```python
from build123d import *

# Parameters (mm, degrees)
SKETCH1_W           = 60
SKETCH1_H           = 28
SKETCH1_R           = 4.25
BOSS_EXTRUDE1_DEPTH = 5
CUT_EXTRUDE1_DEPTH  = 35.583232932
CUT_EXTRUDE2_REACH  = 43.34
SKETCH3_R           = 1.75
FILLET1_R           = 5
FILLET2_R           = 2
SKETCH4_R           = 1.25
BOSS_EXTRUDE2_DEPTH = 3
SKETCH5_W           = 3.75
SKETCH5_H           = 8.5
SKETCH5_W_2         = 9.5
BOSS_EXTRUDE4_DEPTH = 10
SKETCH6_W           = 36
SKETCH6_H           = 8.5
CUT_EXTRUDE3_DEPTH  = 1
SKETCH7_R           = 1.75
CUT_EXTRUDE4_DEPTH  = 45.988887539
SKETCH8_R           = 2.1
CUT_EXTRUDE5_DEPTH  = 4
SKETCH9_R           = 2.1
CUT_EXTRUDE6_DEPTH  = 2
CHAMFER1_SIZE       = 0.5
CUT_EXTRUDE7_REACH  = 46.777
SKETCH10_W          = 2.5
SKETCH10_H          = 8.5
FILLET3_R           = 1.5
FILLET4_R           = 1


with BuildPart() as part:
    # Sketch1 → Boss-Extrude1 (new, symmetric)
    with BuildSketch(Plane.XY):
        Rectangle(SKETCH1_W, SKETCH1_H)
        with Locations((-22, 6)):
            Circle(SKETCH1_R, mode=Mode.SUBTRACT)
        with Locations((22, 6)):
            Circle(SKETCH1_R, mode=Mode.SUBTRACT)
    extrude(amount=BOSS_EXTRUDE1_DEPTH, both=True)

    # Sketch2 → Cut-Extrude1 (cut, through all)
    with BuildSketch(Plane(origin=(0, 0, -5), x_dir=(-1, 0, 0), z_dir=(0, 0, -1))):
        Polygon((8, -6.75), (3, -6.75), (3, 4.25), (4, 4.25), (4, 9.25), (7, 9.25), (7, 4.25), (8, 4.25), align=None)
        Polygon((-8, -6.75), (-8, 4.25), (-7, 4.25), (-7, 9.25), (-4, 9.25), (-4, 4.25), (-3, 4.25), (-3, -6.75), align=None)
    extrude(amount=-CUT_EXTRUDE1_DEPTH, mode=Mode.SUBTRACT)

    # Sketch3 → Cut-Extrude2 (cut, up to next)
    with BuildSketch(Plane(origin=(0, 14, 0), x_dir=(1, 0, 0), z_dir=(0, 1, 0)), mode=Mode.PRIVATE) as cut_extrude2_sk1:
        with Locations(Location((-22, 0, 0), (0, 0, 270))):
            Circle(SKETCH3_R)
    cut_extrude2_tool1 = extrude(cut_extrude2_sk1.sketch, amount=-CUT_EXTRUDE2_REACH, mode=Mode.PRIVATE) & part.part
    # Sketch3 → Cut-Extrude2 (cut, up to next)
    with BuildSketch(Plane(origin=(0, 14, 0), x_dir=(1, 0, 0), z_dir=(0, 1, 0)), mode=Mode.PRIVATE) as cut_extrude2_sk2:
        with Locations(Location((22, 0, 0), (0, 0, 270))):
            Circle(SKETCH3_R)
    cut_extrude2_tool2 = extrude(cut_extrude2_sk2.sketch, amount=-CUT_EXTRUDE2_REACH, mode=Mode.PRIVATE) & part.part
    add(cut_extrude2_tool1.solids().sort_by_distance((-22, 14, 0))[0], mode=Mode.SUBTRACT)
    add(cut_extrude2_tool2.solids().sort_by_distance((22, 14, 0))[0], mode=Mode.SUBTRACT)

    # Fillet1
    fillet1_edges = [part.edges().sort_by_distance(p)[0] for p in [
        (-30, 14, 0),
        (30, 14, 0),
        (30, -14, 0),
        (-30, -14, 0),
    ]]
    fillet(fillet1_edges, radius=FILLET1_R)

    # Fillet2
    # the kernel refuses this fillet: 2 mm, written as the material it adds along each edge
    with BuildSketch(Plane(origin=(-8, 4.25, -5), x_dir=(0, -1, 0), z_dir=(0, 0, 1)), Plane(origin=(3, 4.25, -5), x_dir=(0, -1, 0), z_dir=(0, 0, 1))) as fillet2_piece_1:
        with BuildLine():
            CenterArc((1.732050808, 2), FILLET2_R, 210, 60)
            Line((0, 1), (-0.034641016, 0.98))
            ThreePointArc((-0.034641016, 0.98), (-0.04, 0.5), (-0.04, 0))
            Line((-0.04, 0), (0, -0.04))
            Line((0, -0.04), (1.732050808, -0.04))
            Line((1.732050808, -0.04), (1.732050808, 0))
        make_face()
    extrude(amount=10)
    with BuildSketch(Plane(origin=(-3, 4.25, -5), x_dir=(-1, 0, 0), z_dir=(0, 0, 1)), Plane(origin=(8, 4.25, -5), x_dir=(-1, 0, 0), z_dir=(0, 0, 1))) as fillet2_piece_2:
        with BuildLine():
            CenterArc((2, 1.732050808), FILLET2_R, 180, 60)
            Line((0, 1.732050808), (-0.04, 1.732050808))
            Line((-0.04, 1.732050808), (-0.04, 0))
            Line((-0.04, 0), (0, -0.04))
            ThreePointArc((0, -0.04), (0.5, -0.04), (0.98, -0.034641016))
            Line((0.98, -0.034641016), (1, 0))
        make_face()
    extrude(amount=10)

    # Sketch4 → Boss-Extrude2 (add)
    with BuildSketch(Plane(origin=(0, 0, -5), x_dir=(-1, 0, 0), z_dir=(0, 0, -1))):
        with BuildLine():
            Line((-18, 14), (18, 14))
            Line((18, 14), (18, 29))
            ThreePointArc((18, 29), (17.121320344, 31.121320344), (15, 32))
            Line((15, 32), (-15, 32))
            ThreePointArc((-15, 32), (-17.121320344, 31.121320344), (-18, 29))
            Line((-18, 29), (-18, 14))
        make_face()
        with Locations((-13.85, 22.25)):
            Circle(SKETCH4_R, mode=Mode.SUBTRACT)
        with Locations((13.85, 22.25)):
            Circle(SKETCH4_R, mode=Mode.SUBTRACT)
        with BuildLine():
            Line((-11.65, 28.5), (11.65, 28.5))
            ThreePointArc((11.65, 28.5), (12.003553391, 28.353553391), (12.15, 28))
            Line((12.15, 28), (12.15, 16.5))
            ThreePointArc((12.15, 16.5), (12.003553391, 16.146446609), (11.65, 16))
            Line((11.65, 16), (-11.65, 16))
            ThreePointArc((-11.65, 16), (-12.003553391, 16.146446609), (-12.15, 16.5))
            Line((-12.15, 16.5), (-12.15, 28))
            ThreePointArc((-12.15, 28), (-12.003553391, 28.353553391), (-11.65, 28.5))
        make_face(mode=Mode.SUBTRACT)
    extrude(amount=-BOSS_EXTRUDE2_DEPTH)

    # Sketch5 → Boss-Extrude4 (add)
    with BuildSketch(Plane.XY.offset(5)):
        with Locations((-8.125, -2.5)):
            Rectangle(SKETCH5_W, SKETCH5_H)
        with Locations((0, -2.5)):
            Rectangle(SKETCH5_W_2, SKETCH5_H)
        with Locations((8.125, -2.5)):
            Rectangle(SKETCH5_W, SKETCH5_H)
    extrude(amount=-BOSS_EXTRUDE4_DEPTH)

    # Sketch6 → Cut-Extrude3 (cut)
    with BuildSketch(Plane.XY.offset(5)):
        with Locations((0, -2.5)):
            Rectangle(SKETCH6_W, SKETCH6_H)
    extrude(amount=-CUT_EXTRUDE3_DEPTH, mode=Mode.SUBTRACT)

    # Sketch7 → Cut-Extrude4 (cut, through all)
    with BuildSketch(Plane.XY.offset(5)):
        with Locations((25.5, -9.5)):
            Circle(SKETCH7_R)
        with Locations((-25.5, -9.5)):
            Circle(SKETCH7_R)
        with Locations((-12, 6)):
            Circle(SKETCH7_R)
        with Locations((12, 6)):
            Circle(SKETCH7_R)
    extrude(amount=-CUT_EXTRUDE4_DEPTH, mode=Mode.SUBTRACT)

    # Sketch8 → Cut-Extrude5 (cut)
    with BuildSketch(Plane(origin=(0, 0, 5), x_dir=(-1, 0, 0), z_dir=(0, 0, -1))):
        with Locations((-12, 6)):
            Circle(SKETCH8_R)
        with Locations((-25.5, -9.5)):
            Circle(SKETCH8_R)
        with Locations((25.5, -9.5)):
            Circle(SKETCH8_R)
        with Locations((12, 6)):
            Circle(SKETCH8_R)
    extrude(amount=CUT_EXTRUDE5_DEPTH, mode=Mode.SUBTRACT)

    # Sketch9 → Cut-Extrude6 (cut)
    with BuildSketch(Plane.XZ.offset(-14)):
        with Locations(Location((-22, 0, 0), (0, 0, 270))):
            Circle(SKETCH9_R)
        with Locations(Location((22, 0, 0), (0, 0, 270))):
            Circle(SKETCH9_R)
    extrude(amount=CUT_EXTRUDE6_DEPTH, mode=Mode.SUBTRACT)

    # Chamfer1
    # the kernel refuses this chamfer: 0.5 mm, written as the material it takes off along each edge
    with BuildSketch(Plane(origin=(-25.5, -9.5, 1), x_dir=(1, 0, 0), z_dir=(0, -1, 0))) as chamfer1_piece_1_section:
        Polygon((1.75, -CHAMFER1_SIZE), (1.75 + CHAMFER1_SIZE, 0), (1.75, 0), align=None)
    chamfer1_piece_1 = revolve(axis=Axis((-25.5, -9.5, 1), (0, 0, 1)), mode=Mode.PRIVATE)
    chamfer1_piece_1 = chamfer1_piece_1 & Plane(origin=(-25.5, -9.5, 0.675956313), x_dir=(-1, 0, 0), z_dir=(0, 0, 1)) * Cylinder(2.1, 9, mode=Mode.PRIVATE)
    add(chamfer1_piece_1, mode=Mode.SUBTRACT)
    with BuildSketch(Plane(origin=(25.5, -9.5, 1), x_dir=(1, 0, 0), z_dir=(0, -1, 0))) as chamfer1_piece_2_section:
        Polygon((1.75, -CHAMFER1_SIZE), (1.75 + CHAMFER1_SIZE, 0), (1.75, 0), align=None)
    chamfer1_piece_2 = revolve(axis=Axis((25.5, -9.5, 1), (0, 0, 1)), mode=Mode.PRIVATE)
    chamfer1_piece_2 = chamfer1_piece_2 & Plane(origin=(25.5, -9.5, 0.675956313), x_dir=(-1, 0, 0), z_dir=(0, 0, 1)) * Cylinder(2.1, 9, mode=Mode.PRIVATE)
    add(chamfer1_piece_2, mode=Mode.SUBTRACT)
    with BuildSketch(Plane(origin=(-22, 12, 0), x_dir=(0, 0, 1), z_dir=(-1, 0, 0))) as chamfer1_piece_3_section:
        Polygon((1.75, -CHAMFER1_SIZE), (1.75 + CHAMFER1_SIZE, 0), (1.75, 0), align=None)
    chamfer1_piece_3 = revolve(axis=Axis((-22, 12, 0), (0, 1, 0)), mode=Mode.PRIVATE)
    chamfer1_piece_3 = chamfer1_piece_3 & Plane(origin=(-22, 11.675956313, 0), x_dir=(0, 0, -1), z_dir=(0, 1, 0)) * Cylinder(2.1, 9, mode=Mode.PRIVATE)
    add(chamfer1_piece_3, mode=Mode.SUBTRACT)
    with BuildSketch(Plane(origin=(22, 12, 0), x_dir=(0, 0, 1), z_dir=(-1, 0, 0))) as chamfer1_piece_4_section:
        Polygon((1.75, -CHAMFER1_SIZE), (1.75 + CHAMFER1_SIZE, 0), (1.75, 0), align=None)
    chamfer1_piece_4 = revolve(axis=Axis((22, 12, 0), (0, 1, 0)), mode=Mode.PRIVATE)
    chamfer1_piece_4 = chamfer1_piece_4 & Plane(origin=(22, 11.675956313, 0), x_dir=(0, 0, -1), z_dir=(0, 1, 0)) * Cylinder(2.1, 9, mode=Mode.PRIVATE)
    add(chamfer1_piece_4, mode=Mode.SUBTRACT)
    with BuildSketch(Plane(origin=(-12, 6, 1), x_dir=(1, 0, 0), z_dir=(0, -1, 0))) as chamfer1_piece_5_section:
        Polygon((1.75, -CHAMFER1_SIZE), (1.75 + CHAMFER1_SIZE, 0), (1.75, 0), align=None)
    chamfer1_piece_5 = revolve(axis=Axis((-12, 6, 1), (0, 0, 1)), mode=Mode.PRIVATE)
    chamfer1_piece_5 = chamfer1_piece_5 & Plane(origin=(-12, 6, 0.675956313), x_dir=(-1, 0, 0), z_dir=(0, 0, 1)) * Cylinder(2.1, 9, mode=Mode.PRIVATE)
    add(chamfer1_piece_5, mode=Mode.SUBTRACT)
    with BuildSketch(Plane(origin=(12, 6, 1), x_dir=(1, 0, 0), z_dir=(0, -1, 0))) as chamfer1_piece_6_section:
        Polygon((1.75, -CHAMFER1_SIZE), (1.75 + CHAMFER1_SIZE, 0), (1.75, 0), align=None)
    chamfer1_piece_6 = revolve(axis=Axis((12, 6, 1), (0, 0, 1)), mode=Mode.PRIVATE)
    chamfer1_piece_6 = chamfer1_piece_6 & Plane(origin=(12, 6, 0.675956313), x_dir=(-1, 0, 0), z_dir=(0, 0, 1)) * Cylinder(2.1, 9, mode=Mode.PRIVATE)
    add(chamfer1_piece_6, mode=Mode.SUBTRACT)

    # Sketch10 → Cut-Extrude7 (cut, up to next)
    with BuildSketch(Plane.XY.offset(4), mode=Mode.PRIVATE) as cut_extrude7_sk1:
        with Locations((-16.75, -2.5)):
            Rectangle(SKETCH10_W, SKETCH10_H)
    cut_extrude7_tool1 = extrude(cut_extrude7_sk1.sketch, amount=-CUT_EXTRUDE7_REACH, mode=Mode.PRIVATE) & part.part
    # Sketch10 → Cut-Extrude7 (cut, up to next)
    with BuildSketch(Plane.XY.offset(4), mode=Mode.PRIVATE) as cut_extrude7_sk2:
        with Locations((16.75, -2.5)):
            Rectangle(SKETCH10_W, SKETCH10_H)
    cut_extrude7_tool2 = extrude(cut_extrude7_sk2.sketch, amount=-CUT_EXTRUDE7_REACH, mode=Mode.PRIVATE) & part.part
    add(cut_extrude7_tool1.solids().sort_by_distance((-16.75, -2.5, 4))[0], mode=Mode.SUBTRACT)
    add(cut_extrude7_tool2.solids().sort_by_distance((16.75, -2.5, 4))[0], mode=Mode.SUBTRACT)

    # Fillet3
    fillet3_edges = [part.edges().sort_by_distance(p)[0] for p in [
        (-6.25, 1.75, -0.5),
        (-4.75, 1.75, -0.5),
        (4.75, 1.75, -0.5),
        (6.25, 1.75, -0.5),
        (6.25, -2.5, 4),
        (-6.25, -2.5, 4),
        (-4.75, -2.5, 4),
        (4.75, -2.5, 4),
        (-15.5, -2.5, 4),
        (15.5, -2.5, 4),
    ]]
    fillet(fillet3_edges, radius=FILLET3_R)

    # Fillet4
    fillet4_edges = [part.edges().sort_by_distance(p)[0] for p in [
        (-4, 4.25, 0),
        (-4, 9.25, 0),
        (-7, 9.25, 0),
        (-7, 4.25, 0),
        (7, 4.25, 0),
        (7, 9.25, 0),
        (4, 9.25, 0),
        (4, 4.25, 0),
    ]]
    fillet(fillet4_edges, radius=FILLET4_R)


solid = part.part
```
CAD build for the part. Positions are in the model's coordinates, mm. A direction names the side the tool comes from. Give positions to 0.01 mm unless a question says otherwise; leave off trailing zeros. Write each loop counter-clockwise with the first axis right and the second up, starting at its lowest first coordinate (ties: lowest second). Pieces come first, ordered by that corner, then holes. Notation, with made-up numbers: M -12,45 L 34,45 A21 cw 34,80 Z; hole C 32.5,5 d9. An arc over 180 degrees is marked long. Return JSON: item names as keys, results as strings. Group by question number.
(1) Band-saw the part on B-B (x = 22). Give the cut face in (y, z), and give its area (3 significant figures).
(2) Mould opens along Y. For faces 1 (the face through (0, 32, -4)), 2 (the face through (23.75, -9.42, -2.21)), 3 (the face through (-29, -12, 0)), 4 (the face through (-3.17, 3.32, -0.07)) say: pulls with the +Y half, pulls with the -Y half, needs draft (parallel to the pull), parting line crosses it, or undercut.
(3) Band-saw the part on A-A (y = -2.5). Give the cut face in (x, z).
(4) Flat gauge pins, fed straight in: pin 1 Ø2.5 at (y, z) = (21.5, -4) entering from -X; pin 2 Ø1 at (y, z) = (21.5, -3.5) entering from +X; pin 3 Ø5.5 at (x, y) = (12, 6) entering from -Z; pin 4 Ø8 at (x, y) = (-16.5, 18.5) entering from +Z. Where does each tip first touch, or does it go through?
(5) Drill centre lines: L1, parallel to Y at x = -22, z = -2.5; L2, parallel to X at y = -1, z = 2.75; L3, parallel to Y at x = 12, z = 2.25. Where is each one in solid material? Low to high. Write a range as [from, to].
(6) Band-saw the part on D-D (y = 6). State how many separate pieces and enclosed holes the cut face has, and give its area (3 significant figures).
(7) Band-saw the part on C-C (y = 22.25). Give the cut face in (x, z), and give its area (3 significant figures).
(8) 3-axis set-ups, long thin cutter, end or side, ignore diameter. For faces 5 (the face through (30, 0, 0)), 6 (the face through (3.18, 3.35, -0.07)): which of +Z, -Z, +X, -X, +Y, -Y reach the whole face in a straight line?
Entries:
{
 "1": {"outline": "M -14,-5 L 1.75,-5 L 1.75,5 L -14,5 Z; M 10.25,-5 L 14,-5 L 14,-2.1 L 11.85,-2.1 L 11.5,-1.75 L 10.25,-1.75 Z; M 10.25,1.75 L 11.5,1.75 L 11.85,2.1 L 14,2.1 L 14,5 L 10.25,5 Z", "area": "180 mm^2"},
 "2": {"face 1": "pulls with the +Y half", "face 2": "undercut", "face 3": "pulls with the -Y half", "face 4": "undercut"},
 "3": {"outline": "M -30,-5 L -18,-5 L -18,5 L -30,5 Z; M -15.5,-5 L -6.25,-5 L -6.25,2.5 A1.5 ccw -7.75,4 L -14,4 A1.5 ccw -15.5,2.5 Z; M -4.75,-5 L 4.75,-5 L 4.75,2.5 A1.5 ccw 3.25,4 L -3.25,4 A1.5 ccw -4.75,2.5 Z; M 6.25,-5 L 15.5,-5 L 15.5,2.5 A1.5 ccw 14,4 L 7.75,4 A1.5 ccw 6.25,2.5 Z; M 18,-5 L 30,-5 L 30,5 L 18,5 Z"},
 "4": {"pin 1": "stops at x = -18", "pin 2": "stops at x = 18", "pin 3": "stops at z = -5", "pin 4": "stops at z = -2"},
 "5": {"L1": "y = [-14, 1.75], [10.25, 14]", "L2": "x = [-30, -18], [-15.48, -6.27], [-4.73, 4.73], [6.27, 15.48], [18, 30]", "L3": "y = [-14, 3.9], [8.1, 14]"},
 "6": {"separate pieces": "7", "enclosed holes": "0", "area": "294 mm^2"},
 "7": {"outline": "M -18,-5 L -15.1,-5 L -15.1,-2 L -18,-2 Z; M -12.6,-5 L -12.15,-5 L -12.15,-2 L -12.6,-2 Z; M 12.15,-5 L 12.6,-5 L 12.6,-2 L 12.15,-2 Z; M 15.1,-5 L 18,-5 L 18,-2 L 15.1,-2 Z", "area": "20.1 mm^2"},
 "8": {"face 5": "+Z, -Z, +X, +Y, -Y", "face 6": "+Z, -Z"}
}
